```python
from build123d import *

# Parameters (mm, degrees)
PAD_DEPTH       = 80
PAD_DEPTH_BACK  = 20
SKETCH001_R     = 2.6
SKETCH001_R_2   = 1.6
SKETCH001_R_3   = 0.5
POCKET_DEPTH    = 18.001
SKETCH002_W     = 66.71416
SKETCH002_H     = 42.248775
POCKET001_DEPTH = 13
SKETCH003_R     = 10.65
POCKET002_DEPTH = 30.4
SKETCH004_R     = 10.65
POCKET003_DEPTH = 30.4
POCKET004_DEPTH = 3
FILLET_R        = 5
FILLET001_R     = 1


with BuildPart() as part:
    # Sketch → Pad (new body, two sides)
    with BuildSketch(Plane.XZ) as pad_sk:
        with BuildLine():
            Line((-80, -18), (-80, -13))
            Line((-80, -13), (-20, -13))
            Line((-20, -13), (-20, 0))
            Line((-7, 0), (-20, 0))
            ThreePointArc((-7, 0), (0, -7), (7, 0))
            Line((7, 0), (20, 0))
            Line((20, 0), (20, -18))
            Line((20, -18), (-80, -18))
        make_face()
    extrude(amount=PAD_DEPTH)
    extrude(pad_sk.sketch, amount=-PAD_DEPTH_BACK)

    # Sketch001 → Pocket (cut, through all)
    with BuildSketch(Plane.XY):
        with Locations((-70, 10)):
            Circle(SKETCH001_R)
        with Locations((-30, 10)):
            Circle(SKETCH001_R)
        with Locations((10, 10)):
            Circle(SKETCH001_R)
        with Locations((-15, -5)):
            Circle(SKETCH001_R_2)
        with Locations((-15, -40)):
            Circle(SKETCH001_R_2)
        with Locations((-15, -75)):
            Circle(SKETCH001_R_2)
        with Locations((15, -5)):
            Circle(SKETCH001_R_2)
        with Locations((15, -40)):
            Circle(SKETCH001_R_2)
        with Locations((15, -75)):
            Circle(SKETCH001_R_2)
        with Locations((0, 20)):
            Circle(SKETCH001_R_3)
        Polygon((-80, 0), (-80, -80), (-20, -80), align=None)
    extrude(amount=-POCKET_DEPTH, mode=Mode.SUBTRACT)

    # Sketch002 → Pocket001 (cut)
    with BuildSketch(Plane.XY):
        with Locations((0, 21.124387)):
            Rectangle(SKETCH002_W, SKETCH002_H)
    extrude(amount=-POCKET001_DEPTH, mode=Mode.SUBTRACT)

    # Sketch003 (on DatumPlane) → Pocket002 (cut)
    with BuildSketch(Plane.XZ.offset(5)):
        Circle(SKETCH003_R)
    extrude(amount=POCKET002_DEPTH, mode=Mode.SUBTRACT)

    # Sketch004 (on DatumPlane) → Pocket003 (cut)
    with BuildSketch(Plane.XZ.offset(75)):
        Circle(SKETCH004_R)
    extrude(amount=-POCKET003_DEPTH, mode=Mode.SUBTRACT)

    # Sketch005 (on DatumPlane) → Pocket004 (cut)
    with BuildSketch(Plane.XY.offset(-18)):
        Polygon((-12.25, -6.587713), (-12.25, -3.412287), (-15, -1.824574), (-17.75, -3.412287), (-17.75, -6.587713), (-15, -8.175426), align=None)
        Polygon((17.75, -6.587713), (17.75, -3.412287), (15, -1.824574), (12.25, -3.412287), (12.25, -6.587713), (15, -8.175426), align=None)
        Polygon((-12.25, -41.587713), (-12.25, -38.412287), (-15, -36.824574), (-17.75, -38.412287), (-17.75, -41.587713), (-15, -43.175426), align=None)
        Polygon((17.75, -41.587713), (17.75, -38.412287), (15, -36.824574), (12.25, -38.412287), (12.25, -41.587713), (15, -43.175426), align=None)
        Polygon((-12.25, -76.587713), (-12.25, -73.412287), (-15, -71.824574), (-17.75, -73.412287), (-17.75, -76.587713), (-15, -78.175426), align=None)
        Polygon((17.75, -76.587713), (17.75, -73.412287), (15, -71.824574), (12.25, -73.412287), (12.25, -76.587713), (15, -78.175426), align=None)
    extrude(amount=POCKET004_DEPTH, mode=Mode.SUBTRACT)

    # Fillet
    fillet_edges = [part.edges().sort_by_distance(p)[0] for p in [
        (-80, 20, -15.5),
        (-80, 0, -15.5),
        (20, -80, -9),
        (20, 20, -15.5),
    ]]
    fillet(fillet_edges, radius=FILLET_R)

    # Fillet001
    fillet001_edges = [part.edges().sort_by_distance(p)[0] for p in [
        (-20, -40, -13),
        (0, 0, -13),
    ]]
    fillet(fillet001_edges, radius=FILLET001_R)


solid = part.part
```
The listing builds one solid part. Answer for the finished solid, in the listing's coordinates (mm). A direction names the side the tool comes from. Give positions to 0.01 mm unless a question says otherwise; leave off trailing zeros. Write each loop counter-clockwise with the first axis right and the second up, starting at its lowest first coordinate (ties: lowest second). Pieces come first, ordered by that corner, then holes. Notation, with made-up numbers: M 89.5,-12.75 L 101.5,-12.75 A15 ccw 101.5,-3.75 Z; hole C -3,26 d9. An arc over 180 degrees is marked long. Write each question's results on one line, items separated by ' | '.
Q1. Section B-B, the plane z = -5.5 is taken. Count the separate pieces of the cut face and the enclosed holes in it, then the cut area to 3 significant figures.
Output values:
separate pieces: 2 | enclosed holes: 6 | area: 1,870 mm2
Q2. Section C-C, the plane y = -21 is taken. Write down the section's boundary in (x, z), then the cut area to 3 significant figures.
Output values:
outline: M -64.25,-18 L 20,-18 L 20,0 L 10.65,0 A10.65 cw -10.65,0 L -20,0 L -20,-12 A1 cw -21,-13 L -64.25,-13 Z | area: 763 mm2
Q3. Flat-ended cylindrical pins translate along their axes: P1, Ø1.6, axis at x = 16, y = -5, coming from the -Z side; P2, Ø3.5, axis at y = -39.5, z = -17, coming from the -X side; P3, Ø1.5, axis at y = -5.5, z = -16, coming from the -X side. Find the tip coordinate at first contact, or state that the pin passes through.
Output values:
P1: z = -15 | P2: x = -51.69 | P3: x = -76.44
Q4. Section D-D, the plane x = -39.5 is taken. Write down the section's boundary in (y, z).
Output values:
outline: M -54,-18 L 20,-18 L 20,-13 L -54,-13 Z
Q5. Consider L1, parallel to Y at x = -15, z = -5.5; L2, parallel to Y at x = 8.5, z = -5; L3, parallel to X at y = -2.5, z = -15.5 (3 decimals). Determine where each line is inside the solid, lowest interval first. Write a range as from..to.
Output values:
L1: -80..-76.6, -73.4..-41.6, -38.4..-6.6, -3.4..0 | L2: -80..-75, -44.6..-35.4, -5..0 | L3: -78.125..-16.17, -13.83..13.83, 16.17..20
Q6. For a pull along Y with two mould halves and no side action, classify faces 4 (the flat face through (-49.1, -41.2, -15.6)), 5 (the cylindrical face through (0, -40, -7)), 6 (the flat face through (-12.25, -75, -17)) as released by +Y, released by -Y, zero draft, split by the parting line, or undercut.
Output values:
face 4: released by -Y | face 5: zero draft | face 6: undercut
Q7. A tool of negligible diameter and unlimited length cuts with its end or side. For faces 1 (the cylindrical face through (0, -78, -7)), 2 (the flat face through (-13.606, -2.63, -16.521)), 3 (the flat face through (-0.3, 0, -7.2)), from which of +Z, -Z, +X, -X, +Y, -Y can it reach the whole face along a straight path? Write none if from no direction.
Output values:
face 1: +Z, +Y, -Y | face 2: -Z | face 3: +Z, +X, -X, +Y
Q8. Section A-A, the plane y = 10 is taken. Write down the section's boundary in (x, z).
Output values:
outline: M -80,-18 L -72.6,-18 L -72.6,-13 L -80,-13 Z; M -67.4,-18 L -32.6,-18 L -32.6,-13 L -67.4,-13 Z; M -27.4,-18 L 7.4,-18 L 7.4,-13 L -27.4,-13 Z; M 12.6,-18 L 20,-18 L 20,-13 L 12.6,-13 Z
